Source: CAD feature listing. Evaluate the final solid. Frame: model axes, mm. Coordinates: 2 decimals unless noted, no trailing zeros. Loops run counter-clockwise (first coordinate to the right, second up) from the corner with the lowest first, then second, coordinate; pieces in that order, holes last. Notation, with made-up numbers: M -16,69 L 30,69 A21 ccw 30,103 Z; hole C 60.5,8.5 d1. An arc over 180 degrees is marked long. One line per question, with ' | ' between items. Start each with the question number.
1. Section query A-A, the plane z = 0.55. State how many separate pieces and enclosed holes the cut face has, and give its area (3 significant figures).
2. Ray query, probe 1 along X at (y, z) = (4.25, 1.1) (3 decimals); probe 2 along X at (y, z) = (3.25, 1.4); probe 3 along Y at (x, z) = (6.5, 1.4). Return the intervals inside material, ascending.
3. Pin query (flat end, axial travel): P1, Ø0.9, axis at x = 89.789, y = 0, coming from the +Z side. Return the tip coordinate at first contact, or that it passes through.
4. Section query B-B, the plane x = 82.5. Output: boundary loops of the cut face in (y, z), and give its area (3 significant figures).
5. Mould query, pull axis X, two halves, no side actions, for faces 1 (the cylindrical face through (9.76, -3.05, 0.79)), 2 (the flat face through (5, -5.08, 1)), 3 (the cylindrical face through (24.244, 0.033, 0.789)), 4 (the flat face through (1.27, 0, 1)). Classes: pulls with the +X half, pulls with the -X half, needs draft (parallel to the pull), parting line crosses it, or undercut.
```python
from build123d import *

# Parameters (mm, degrees)
EXTRUDE_1_OUTLINE_R = 0.325
EXTRUDE_1_DEPTH     = 1.6
SKETCH_1_R          = 0.635
SKETCH_1_R_2        = 0.750616105
CUT_EXTRUDE_1_DEPTH = 92.214625368


# Read off the part's stored shape, not the designer's step: 凸台-拉伸1
with BuildPart() as part:
    # 凸台-拉伸1 outline → 凸台-拉伸1 (new body)
    with BuildSketch(Plane.XY):
        with BuildLine():
            Line((81.153, -5.08), (81.534, -4.699))
            Line((81.534, -4.699), (81.534, -4.064))
            ThreePointArc((81.534, -4.064), (82.55, -3.048), (83.566, -4.064))
            Line((83.566, -4.064), (83.566, -4.699))
            Line((83.566, -4.699), (83.947, -5.08))
            Line((83.947, -5.08), (90.678, -5.08))
            Line((90.678, -5.08), (91.059, -4.699))
            Line((91.059, -4.699), (91.059, 0))
            Line((91.059, 0), (1.27, 0))
            Line((1.27, 0), (1.27, -4.699))
            Line((1.27, -4.699), (1.651, -5.08))
            Line((1.651, -5.08), (8.382, -5.08))
            Line((8.382, -5.08), (8.763, -4.699))
            Line((8.763, -4.699), (8.763, -4.064))
            ThreePointArc((8.763, -4.064), (9.779, -3.048), (10.795, -4.064))
            Line((10.795, -4.064), (10.795, -4.699))
            Line((10.795, -4.699), (11.176, -5.08))
            Line((11.176, -5.08), (81.153, -5.08))
        make_face()
        with BuildLine():
            Line((2.728, -4.02), (3.348, -4.02))
            ThreePointArc((3.348, -4.02), (3.648, -4.32), (3.348, -4.62))
            Line((3.348, -4.62), (2.728, -4.62))
            ThreePointArc((2.728, -4.62), (2.428, -4.32), (2.728, -4.02))
        make_face(mode=Mode.SUBTRACT)
        with BuildLine():
            Line((7.763, -4.62), (6.663, -4.62))
            ThreePointArc((6.663, -4.62), (6.363, -4.32), (6.663, -4.02))
            Line((6.663, -4.02), (7.763, -4.02))
            ThreePointArc((7.763, -4.02), (8.063, -4.32), (7.763, -4.62))
        make_face(mode=Mode.SUBTRACT)
        with Locations((6.683, -2.8687)):
            Circle(EXTRUDE_1_OUTLINE_R, mode=Mode.SUBTRACT)
    extrude_1 = extrude(amount=EXTRUDE_1_DEPTH)

    # 镜向1: 凸台-拉伸1 across plane
    add(extrude_1.mirror(Plane(origin=(0, 0, 1.6), x_dir=(0, 0, 1), z_dir=(0, 1, 0))))

    # 草图1 → 切除-拉伸1 (cut, through all)
    with BuildSketch(Plane.XY):
        with Locations((19.914, 0)):
            Circle(SKETCH_1_R)
        with Locations((24.994, 0)):
            Circle(SKETCH_1_R_2)
        with Locations((29.414, 0)):
            Circle(SKETCH_1_R_2)
        with Locations((34.494, 0)):
            Circle(SKETCH_1_R_2)
        with Locations((89.789, 0)):
            Circle(SKETCH_1_R_2)
        with Locations((84.709, 0)):
            Circle(SKETCH_1_R_2)
    extrude(amount=CUT_EXTRUDE_1_DEPTH, mode=Mode.SUBTRACT)


solid = part.part
```
Taken from the geometry:
1) separate pieces: 1 | enclosed holes: 12 | area: 883 mm^2
2) probe 1: 1.27 to 2.436, 3.64 to 6.371, 8.055 to 8.763, 10.795 to 81.534, 83.566 to 91.059 | probe 2: 1.27 to 9.17, 10.39 to 81.94, 83.16 to 91.06 | probe 3: -5.08 to -4.57, -4.07 to -3.14, -2.6 to 2.6, 3.14 to 4.07, 4.57 to 5.08
3) P1: through
4) outline: M -3.05,0 L 3.05,0 L 3.05,1.6 L -3.05,1.6 Z | area: 9.76 mm^2
5) face 1: undercut | face 2: needs draft | face 3: undercut | face 4: pulls with the -X half
